```python
from build123d import *

# Parameters (mm, degrees)
SKETCH_1_R          = 65
SKETCH_1_R_2        = 60
EXTRUDE_1_DEPTH     = 150
SKETCH_2_R          = 85
SKETCH_2_R_2        = 3
SKETCH_2_R_3        = 65
EXTRUDE_2_DEPTH     = 8
SKETCH_3_R          = 70
SKETCH_3_R_2        = 65
CUT_EXTRUDE_1_DEPTH = 3


with BuildPart() as part:
    # 草图1 → 凸台-拉伸1 (new, symmetric)
    with BuildSketch(Plane.XY):
        Circle(SKETCH_1_R)
        Circle(SKETCH_1_R_2, mode=Mode.SUBTRACT)
    extrude(amount=EXTRUDE_1_DEPTH, both=True)

    # 草图2 → 凸台-拉伸2 (add)
    with BuildSketch(Plane.XY.offset(150)):
        Circle(SKETCH_2_R)
        with Locations((0, 75)):
            Circle(SKETCH_2_R_2, mode=Mode.SUBTRACT)
        with Locations((64.951905284, 37.5)):
            Circle(SKETCH_2_R_2, mode=Mode.SUBTRACT)
        with Locations((64.951905284, -37.5)):
            Circle(SKETCH_2_R_2, mode=Mode.SUBTRACT)
        with Locations((0, -75)):
            Circle(SKETCH_2_R_2, mode=Mode.SUBTRACT)
        with Locations((-64.951905284, -37.5)):
            Circle(SKETCH_2_R_2, mode=Mode.SUBTRACT)
        with Locations((-64.951905284, 37.5)):
            Circle(SKETCH_2_R_2, mode=Mode.SUBTRACT)
        Circle(SKETCH_2_R_3, mode=Mode.SUBTRACT)
    extrude_2 = extrude(amount=-EXTRUDE_2_DEPTH)

    # 草图3 → 切除-拉伸1 (cut)
    with BuildSketch(Plane.XY.offset(150)):
        Circle(SKETCH_3_R)
        Circle(SKETCH_3_R_2, mode=Mode.SUBTRACT)
    cut_extrude_1 = extrude(amount=-CUT_EXTRUDE_1_DEPTH, mode=Mode.SUBTRACT)

    # 镜向1: 凸台-拉伸2, 切除-拉伸1 across plane
    add(extrude_2.mirror(Plane.XY))
    add(cut_extrude_1.mirror(Plane.XY), mode=Mode.SUBTRACT)


solid = part.part
```
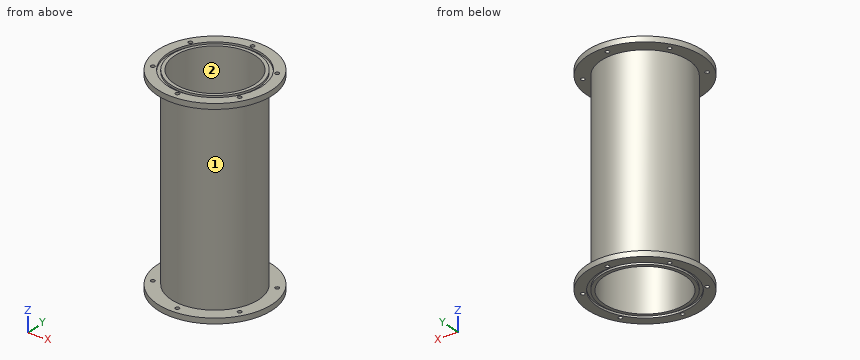
Can you work these out from the model? Positions are in its coordinate system, mm. Face numbers are marked on the shaded views. Give positions to 0.01 mm unless a question says otherwise; leave off trailing zeros. Loops run counter-clockwise (first coordinate to the right, second up) from the corner with the lowest first, then second, coordinate; pieces in that order, holes last. Notation, with made-up numbers: M 6.5,70 L 17.5,70 A11 cw 17.5,81 Z; hole C 69,40 d1. An arc over 180 degrees is marked long. Use CSV: the item, a comma, the result in double quotes. Start each with the question number.
1. If I drill on L1, parallel to Z at x = -46.5, y = 56.5; L2, parallel to X at y = 37, z = 78; L3, parallel to Y at x = 20.5, z = -4, over which ranges is the centre line in solid material (lowest first)?
2. For P1, Ø10, axis at y = -28.5, z = -17.5, coming from the -X side; P2, Ø5.5, axis at x = 64.95, y = 37.5, coming from the +Z side; P3, Ø1, axis at x = 10.5, y = -67.5, coming from the +Z side; P4, Ø1.5, axis at y = 10.5, z = -33, coming from the -X side, each with a flat end and sliding along its axis, tell me the tip position at first contact or that it passes through.
3. If we mould it in two halves opening along Z, with no side actions, what happens to the marked faces 1 and 2? For each: released by +Z, released by -Z, zero draft, split by the parting line, or undercut.
4. Imagine slicing it at C-C, the plane z = 50. Write out the boundary of the cut face in (x, y).
Response values:
1,L1,"-150 to -142, 142 to 150"
1,L2,"-53.44 to -47.23, 47.23 to 53.44"
1,L3,"-61.68 to -56.39, 56.39 to 61.68"
2,P1,"x = -60.6"
2,P2,"through"
2,P3,"z = 147"
2,P4,"x = -64.26"
3,face 1,"undercut"
3,face 2,"zero draft"
4,outline,"C 0,0 d130; hole C 0,0 d120"
